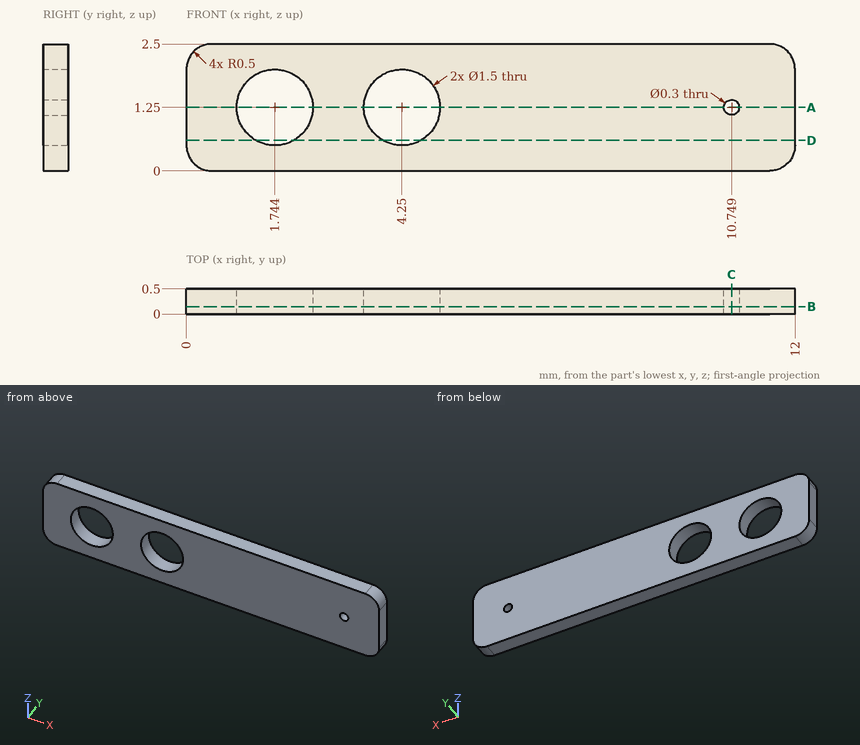
Print and shaded views of the part. All mm, measured from the part's lowest x, y and z. Give positions to 0.01 mm unless a question says otherwise; leave off trailing zeros. Write each loop counter-clockwise with the first axis right and the second up, starting at its lowest first coordinate (ties: lowest second). Pieces come first, ordered by that corner, then holes. Notation, with made-up numbers: (11.25, 89.5) -> (48.25, 89.5) arc R7 ccw to (48.25, 96.5) -> close; hole circle Ø2 at (47.5, 41). An arc over 180 degrees is marked (long way). Use CSV: the item, a comma, the result in double quotes. Start each with the question number.
1) Drill centre lines: L1, parallel to X at y = 0.4, z = 1.25; L2, parallel to X at y = 0.3, z = 1.6 (1 decimal); L3, parallel to Z at x = 4.25, y = 0.35. Where is each one in solid material? Low to high.
2) Cut at A-A on z = 1.25. List the corners of the cut face in (x, y).
3) Cut at C-C on x = 10.75. List the corners of the cut face in (y, z).
4) Cut at D-D on z = 0.6. List the corners of the cut face in (x, y) (1 decimal).
5) Cut at B-B on y = 0.15. List the corners of the cut face in (x, z).
Final values:
1,L1,"x = 0 to 0.99, 2.49 to 3.5, 5 to 10.6, 10.9 to 12"
1,L2,"x = 0 to 1.1, 2.4 to 3.6, 4.9 to 12"
1,L3,"z = 0 to 0.5, 2 to 2.5"
2,outline,"(0, 0) -> (0.99, 0) -> (0.99, 0.5) -> (0, 0.5) -> close; (2.49, 0) -> (3.5, 0) -> (3.5, 0.5) -> (2.49, 0.5) -> close; (5, 0) -> (10.6, 0) -> (10.6, 0.5) -> (5, 0.5) -> close; (10.9, 0) -> (12, 0) -> (12, 0.5) -> (10.9, 0.5) -> close"
3,outline,"(0, 0) -> (0.5, 0) -> (0.5, 1.1) -> (0, 1.1) -> close; (0, 1.4) -> (0.5, 1.4) -> (0.5, 2.5) -> (0, 2.5) -> close"
4,outline,"(0, 0) -> (1.4, 0) -> (1.4, 0.5) -> (0, 0.5) -> close; (2.1, 0) -> (3.9, 0) -> (3.9, 0.5) -> (2.1, 0.5) -> close; (4.6, 0) -> (12, 0) -> (12, 0.5) -> (4.6, 0.5) -> close"
5,outline,"(0, 0.5) arc R0.5 ccw to (0.5, 0) -> (11.5, 0) arc R0.5 ccw to (12, 0.5) -> (12, 2) arc R0.5 ccw to (11.5, 2.5) -> (0.5, 2.5) arc R0.5 ccw to (0, 2) -> close; hole circle Ø1.5 at (1.74, 1.25); hole circle Ø1.5 at (4.25, 1.25); hole circle Ø0.3 at (10.75, 1.25)"
